Build history of the part. All positions in model axes, mm. A direction names the side the tool comes from. Give positions to 0.01 mm unless a question says otherwise; leave off trailing zeros. Loops run counter-clockwise (first coordinate to the right, second up) from the corner with the lowest first, then second, coordinate; pieces in that order, holes last. Notation, with made-up numbers: M 72.25,25.25 L 76.25,25.25 A16 ccw 76.25,34.25 Z; hole C 60.5,-17 d4. An arc over 180 degrees is marked long. Answer as a JSON object with one key per item and string values. Group by question number.
1. Slice it at B-B (y = 302.5). List the corners of the cut face in (x, z), then the cut area to 3 significant figures.
2. Drill centre lines: line 1 along X through (y, z) = (445, -17.25); line 2 along X through (y, z) = (532.6, -1); line 3 along Z through (x, y) = (8.5, 85.5). Where is each one in solid material? Low to high. Write a range as [from, to].
3. 3-axis set-ups, long thin cutter, end or side, ignore diameter. For faces 1 (the face through (18, 558.8, -9)), 2 (the face through (17.462, 275, -9)): which of +Z, -Z, +X, -X, +Y, -Y reach the whole face in a straight line?
4. Mould opens along X. For faces 3 (the face through (9, 275, -19.05)), 4 (the face through (19.05, 275, -9)), 5 (the face through (1.588, 275, -9)) say: released by +X, released by -X, zero draft, split by the parting line, or undercut.
from build123d import *

# Parameters (mm, degrees)
SKETCH1_W           = 19.05
SKETCH1_H           = 19.05
SKETCH1_W_2         = 15.875
SKETCH1_H_2         = 15.875
BOSS_EXTRUDE1_DEPTH = 914.4
SKETCH4_R           = 6.35
CUT_EXTRUDE3_DEPTH  = 20.05
SKETCH5_OUTSIDE_W   = 204.01
SKETCH5_OUTSIDE_H   = 1099.36
SKETCH5_OUTSIDE_W_2 = 19.05
SKETCH5_OUTSIDE_H_2 = 558.8
CUT_EXTRUDE4_DEPTH  = 20.05
SKETCH6_R           = 2.75
CUT_EXTRUDE5_DEPTH  = 20.05


with BuildPart() as part:
    # Sketch1 → Boss-Extrude1 (new body)
    with BuildSketch(Plane(origin=(0, 0, 0), x_dir=(1, 0, 0), z_dir=(0, 1, 0))):
        with Locations((9.525, 9.525)):
            Rectangle(SKETCH1_W, SKETCH1_H)
        with Locations((9.525, 9.525)):
            Rectangle(SKETCH1_W_2, SKETCH1_H_2, mode=Mode.SUBTRACT)
    extrude(amount=BOSS_EXTRUDE1_DEPTH)

    # Sketch4 → Cut-Extrude3 (cut, through all)
    with BuildSketch(Plane(origin=(19.05, 0, 0), x_dir=(0, 0, -1), z_dir=(1, 0, 0))):
        with Locations((9.525, 20)):
            Circle(SKETCH4_R)
    extrude(amount=-CUT_EXTRUDE3_DEPTH, mode=Mode.SUBTRACT)

    # Sketch5 outside → Cut-Extrude4 (cut, through all)
    with BuildSketch(Plane.XY):
        with Locations((9.525, 457.2)):
            Rectangle(SKETCH5_OUTSIDE_W, SKETCH5_OUTSIDE_H)
        with Locations((9.525, 279.4)):
            Rectangle(SKETCH5_OUTSIDE_W_2, SKETCH5_OUTSIDE_H_2, mode=Mode.SUBTRACT)
    extrude(amount=-CUT_EXTRUDE4_DEPTH, mode=Mode.SUBTRACT)

    # Sketch6 → Cut-Extrude5 (cut, through all)
    with BuildSketch(Plane(origin=(0, 0, -19.05), x_dir=(-1, 0, 0), z_dir=(0, 0, -1))):
        with Locations((-9.53, 532.6)):
            Circle(SKETCH6_R)
        with Locations((-9.53, 502.6)):
            Circle(SKETCH6_R)
    extrude(amount=-CUT_EXTRUDE5_DEPTH, mode=Mode.SUBTRACT)


solid = part.part
Established:
{
 "1": {"outline": "M 0,-19.05 L 19.05,-19.05 L 19.05,0 L 0,0 Z; hole M 1.59,-17.46 L 17.46,-17.46 L 17.46,-1.59 L 1.59,-1.59 Z", "area": "111 mm^2"},
 "2": {"line 1": "x = [0, 1.59], [17.46, 19.05]", "line 2": "x = [0, 6.78], [12.28, 19.05]", "line 3": "z = [-19.05, -17.46], [-1.59, 0]"},
 "3": {"face 1": "+Z, -Z, +X, -X, +Y", "face 2": "+Y, -Y"},
 "4": {"face 3": "zero draft", "face 4": "released by +X", "face 5": "undercut"}
}
